Can you work these out from the model? Positions are in its coordinate system, mm. Give positions to 0.01 mm unless a question says otherwise; leave off trailing zeros. Loops run counter-clockwise (first coordinate to the right, second up) from the corner with the lowest first, then second, coordinate; pieces in that order, holes last. Notation, with made-up numbers: (-20, -35.5) - (9, -35.5) arc R13 cw to (9, -15.5) - close; hole circle Ø9 at (16.5, 39.25). An arc over 180 degrees is marked (long way). Answer as a JSON object with one key per item and string values. Group by question number.
Item 1: Will this pin go through, and if not, where does the flat tip stop? pin 1 (2 mm diameter, centred on x = -132, y = 5.5, fed in from +Z).
Item 2: Suppose I cut it at D-D on x = -92. Write out the boundary of the cut face in (y, z), and give its area (3 significant figures).
Item 3: Please list where these lines run through material, in increasing order: L1, parallel to Y at x = -158, z = 2.8; L2, parallel to Y at x = -92, z = 1.1; L3, parallel to Y at x = -30.5, z = 3.4.
Item 4: Suppose I cut it at C-C on z = 3.55. Count the separate pieces of the cut face and the enclosed holes in it, and give its area (3 significant figures).
Item 5: Suppose I cut it at B-B on x = -132. Write out the boundary of the cut face in (y, z), and give its area (3 significant figures).
Item 6: Suppose I cut it at A-A on y = 63.5. Write out the boundary of the cut face in (x, z).
Autodesk Inventor part; units mm, degrees
ref_plane "YZ Plane" through (0, 0, 0) normal (1, 0, 0) x (0, 1, 0)
ref_plane "XZ Plane" through (0, 0, 0) normal (0, 1, 0) x (-1, 0, 0)
ref_plane "XY Plane" through (0, 0, 0) normal (0, 0, 1) x (1, 0, 0)
sketch "Эскиз1" plane through (0, 0, 0) normal (0, 0, 1) x (1, 0, 0)
  line L0 (0, 0) -> (-184, 0)
  line L1 (-184, 0) -> (-184, 90)
  line L2 (-184, 90) -> (0, 90)
  line L3 (0, 90) -> (0, 0)
  dimension "d0" = 184
  dimension "d1" = 90
extrude "Выдавливание1" add sketch "Эскиз1" along normal blind 5
sketch "Эскиз2" plane through (0, 0, 5) normal (0, 0, 1) x (1, 0, 0)
  line L0 (0, 90) -> (-184, 90)
  line L1 (-26, 45) -> (-26, 56)
  line L2 (-26, 56) -> (-158, 56)
  line L3 (-158, 56) -> (-158, 34)
  line L4 (-158, 34) -> (-26, 34)
  line L5 (-26, 34) -> (-26, 56)
  circle A0 centre (-158, 56) radius 1.75
  circle A1 centre (-26, 56) radius 1.75
  circle A2 centre (-26, 34) radius 1.75
  circle A3 centre (-158, 34) radius 1.75
  point P0 (0, 0)
  dimension "d43" = 11
  dimension "d44" = 132
  dimension "d45" = 22
  dimension "d46" = 3.5
  dimension "d47" = 3.5
  dimension "d48" = 3.5
  dimension "d49" = 3.5
extrude "Выдавливание2" cut sketch "Эскиз2" against normal blind 5 contours A1 L2 L1 | L1 L2 A1 | A2 L4 L5 | L5 L4 A2 | A0 L3 L2 | L2 L3 A0 | A3 L3 L4 | L4 L3 A3
sketch "Эскиз8" plane through (0, 0, 5) normal (0, 0, 1) x (1, 0, 0)
  line L0 (-184, 0) -> (-184, 90)
  line L1 (-184, 0) -> (-92, 0)
  line L2 (0, 0) -> (-184, 0)
  line L3 (-92, 0) -> (-92, 10)
  line L4 (-92, 10) -> (-92, 80)
  circle A0 centre (-92, 80) radius 1.75
  circle A1 centre (-92, 10) radius 1.75
  dimension "d52" = 92
  dimension "d53" = 10
  dimension "d54" = 70
  dimension "d55" = 3.5
  dimension "d56" = 3.5
extrude "Выдавливание3" cut sketch "Эскиз8" against normal blind 5
sketch "Эскиз9" plane through (0, 0, 5) normal (0, 0, 1) x (1, 0, 0)
  line L0 (0, 90) -> (0, 85)
  line L1 (0, 90) -> (0, 0)
  line L2 (-60, 85) -> (-60, 5)
  line L3 (-60, 5) -> (0, 5)
  line L4 (0, 5) -> (0, 85)
  line L5 (-184, 90) -> (-184, 87.5)
  line L6 (-184, 0) -> (-184, 90)
  line L7 (-184, 0) -> (-184, 2.5)
  line L8 (-129, 87.5) -> (-129, 2.5)
  line L9 (-129, 2.5) -> (-184, 2.5)
  line L10 (-184, 2.5) -> (-184, 87.5)
  line L11 (-60, 77) -> (-129, 77)
  line L12 (-129, 87.5) -> (-129, 63.5)
  line L13 (-129, 63.5) -> (-132, 63.5)
  circle A0 centre (-132, 63.5) radius 1.75
  circle A1 centre (-180.5, 63.5) radius 1.75
  circle A2 centre (-132, 5.5) radius 1.75
  circle A3 centre (-180.5, 5.5) radius 1.75
  line L14 (-180.5, 63.5) -> (-180.5, 5.5)
  line L15 (-180.5, 5.5) -> (-132, 5.5)
  line L16 (-132, 5.5) -> (-132, 63.5)
  line L17 (-60, 5) -> (-30.5, 5)
  line L18 (-30.5, 5) -> (-30.5, 16)
  circle A4 centre (-30.5, 16) radius 1.75
  line L19 (-30.5, 16) -> (-30.5, 71.5)
  circle A5 centre (-30.5, 71.5) radius 1.75
  dimension "d61" = 5
  dimension "d62" = 60
  dimension "d63" = 80
  dimension "d64" = 2.5
  dimension "d65" = 2.5
  dimension "d66" = 55
  dimension "d67" = 85
  dimension "d69" = 69
  dimension "d70" = 24
  dimension "d71" = 3
  dimension "d72" = 3.5
  dimension "d75" = 3.5
  dimension "d76" = 3.5
  dimension "d77" = 3.5
  dimension "d78" = 58
  dimension "d79" = 48.5
  dimension "d80" = 29.5
  dimension "d81" = 11
  dimension "d82" = 3.5
  dimension "d83" = 55.5
  dimension "d84" = 3.5
extrude "Выдавливание4" cut sketch "Эскиз9" against normal blind 5
sketch "Эскиз10" plane through (0, 0, 5) normal (0, 0, 1) x (1, 0, 0)
  line L0 (0, 0) -> (-184, 0)
  circle A0 centre (-92, 45) radius 10
  dimension "d89" = 20
extrude "Выдавливание5" cut sketch "Эскиз10" against normal blind 5
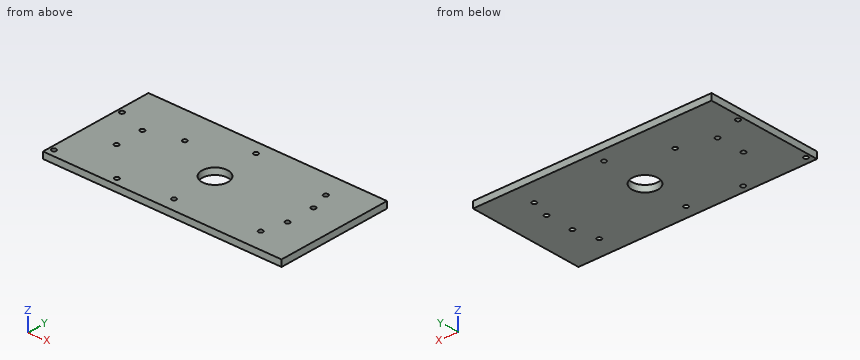
Worked out:
{
 "1": {"pin 1": "passes through"},
 "2": {"outline": "(0, 0) - (8.25, 0) - (8.25, 5) - (0, 5) - close; (11.75, 0) - (35, 0) - (35, 5) - (11.75, 5) - close; (55, 0) - (78.25, 0) - (78.25, 5) - (55, 5) - close; (81.75, 0) - (90, 0) - (90, 5) - (81.75, 5) - close", "area": "315 mm2"},
 "3": {"L1": "y = 0 to 32.25, 35.75 to 54.25, 57.75 to 90", "L2": "y = 0 to 8.25, 11.75 to 35, 55 to 78.25, 81.75 to 90", "L3": "y = 0 to 14.25, 17.75 to 69.75, 73.25 to 90"},
 "4": {"separate pieces": "1", "enclosed holes": "13", "area": "16,100 mm2"},
 "5": {"outline": "(0, 0) - (3.75, 0) - (3.75, 5) - (0, 5) - close; (7.25, 0) - (61.75, 0) - (61.75, 5) - (7.25, 5) - close; (65.25, 0) - (90, 0) - (90, 5) - (65.25, 5) - close", "area": "415 mm2"},
 "6": {"outline": "(-184, 0) - (-182.25, 0) - (-182.25, 5) - (-184, 5) - close; (-178.75, 0) - (-133.75, 0) - (-133.75, 5) - (-178.75, 5) - close; (-130.25, 0) - (0, 0) - (0, 5) - (-130.25, 5) - close"}
}
